from build123d import *

# Parameters (mm, degrees)
SKETCH1_W           = 300
SKETCH1_H           = 170
BOSS_EXTRUDE1_DEPTH = 12
SKETCH2_R           = 4
CUT_EXTRUDE1_DEPTH  = 13
SKETCH4_R           = 4
CUT_EXTRUDE2_DEPTH  = 13
SKETCH5_R           = 4
CUT_EXTRUDE3_DEPTH  = 13
SKETCH6_W           = 46.5
SKETCH6_H           = 93
SKETCH6_W_2         = 80
SKETCH6_H_2         = 45
SKETCH6_W_3         = 64
SKETCH6_H_3         = 67.5
SKETCH6_W_4         = 23.5
SKETCH6_H_4         = 65.5
CUT_EXTRUDE4_DEPTH  = 13
FILLET1_R           = 10


with BuildPart() as part:
    # Sketch1 → Boss-Extrude1 (new body)
    with BuildSketch(Plane(origin=(0, 0, 0), x_dir=(1, 0, 0), z_dir=(0, 1, 0))):
        Rectangle(SKETCH1_W, SKETCH1_H)
    extrude(amount=BOSS_EXTRUDE1_DEPTH)

    # Sketch2 → Cut-Extrude1 (cut, through all)
    with BuildSketch(Plane(origin=(0, 12, 0), x_dir=(1, 0, 0), z_dir=(0, 1, 0))):
        with Locations((-135, 65)):
            Circle(SKETCH2_R)
        with Locations((-135, 23)):
            Circle(SKETCH2_R)
        with Locations((-135, -19)):
            Circle(SKETCH2_R)
        with Locations((-135, -61)):
            Circle(SKETCH2_R)
        with Locations((-135, -103)):
            Circle(SKETCH2_R)
        with Locations((-135, -145)):
            Circle(SKETCH2_R)
    cut_extrude1 = extrude(amount=-CUT_EXTRUDE1_DEPTH, mode=Mode.SUBTRACT)

    # Mirror1: Cut-Extrude1 across plane
    add(cut_extrude1.mirror(Plane(origin=(0, 0, 0), x_dir=(0, 0, 1), z_dir=(1, 0, 0))), mode=Mode.SUBTRACT)

    # Sketch4 → Cut-Extrude2 (cut, through all)
    with BuildSketch(Plane(origin=(0, 12, 0), x_dir=(1, 0, 0), z_dir=(0, 1, 0))):
        with Locations((-110, 65)):
            Circle(SKETCH4_R)
        with Locations((-10, 65)):
            Circle(SKETCH4_R)
        with Locations((-110, 40)):
            Circle(SKETCH4_R)
        with Locations((-10, 40)):
            Circle(SKETCH4_R)
        with Locations((46, 65)):
            Circle(SKETCH4_R)
        with Locations((46, 15)):
            Circle(SKETCH4_R)
    extrude(amount=-CUT_EXTRUDE2_DEPTH, mode=Mode.SUBTRACT)

    # Sketch5 → Cut-Extrude3 (cut, through all)
    with BuildSketch(Plane(origin=(0, 12, 0), x_dir=(1, 0, 0), z_dir=(0, 1, 0))):
        with Locations((-60, -20)):
            Circle(SKETCH5_R)
        with Locations((-60, -50)):
            Circle(SKETCH5_R)
        with Locations((84, -20)):
            Circle(SKETCH5_R)
        with Locations((84, -50)):
            Circle(SKETCH5_R)
    extrude(amount=-CUT_EXTRUDE3_DEPTH, mode=Mode.SUBTRACT)

    # Sketch6 → Cut-Extrude4 (cut, through all)
    with BuildSketch(Plane(origin=(0, 12, 0), x_dir=(1, 0, 0), z_dir=(0, 1, 0))):
        with Locations((-100.75, -26.5)):
            Rectangle(SKETCH6_W, SKETCH6_H)
        Polygon((27.5, 20), (-42.5, 20), (-42.5, -73), (66.5, -73), (66.5, -7.5), (27.5, -7.5), align=None)
        with Locations((-60, 52.5)):
            Rectangle(SKETCH6_W_2, SKETCH6_H_2)
        with Locations((93, 41.25)):
            Rectangle(SKETCH6_W_3, SKETCH6_H_3)
        with Locations((113.25, -40.25)):
            Rectangle(SKETCH6_W_4, SKETCH6_H_4)
    extrude(amount=-CUT_EXTRUDE4_DEPTH, mode=Mode.SUBTRACT)

    # Fillet1
    fillet1_edges = [part.edges().sort_by_distance(p)[0] for p in [
        (-42.5, 6, 73),
        (-42.5, 6, -20),
        (27.5, 6, -20),
        (27.5, 6, 7.5),
        (66.5, 6, 7.5),
        (66.5, 6, 73),
        (-20, 6, -75),
        (-20, 6, -30),
        (-100, 6, -30),
        (-100, 6, -75),
        (125, 6, -75),
        (125, 6, -7.5),
        (61, 6, -7.5),
        (61, 6, -75),
        (125, 6, 7.5),
        (125, 6, 73),
        (101.5, 6, 73),
        (101.5, 6, 7.5),
        (-124, 6, 73),
        (-124, 6, -20),
        (-77.5, 6, -20),
        (-77.5, 6, 73),
    ]]
    fillet(fillet1_edges, radius=FILLET1_R)


solid = part.part
Verification items for the finished model (mm, model axes). Give positions to 0.01 mm unless a question says otherwise; leave off trailing zeros. Write each loop counter-clockwise with the first axis right and the second up, starting at its lowest first coordinate (ties: lowest second). Pieces come first, ordered by that corner, then holes.
(1) Cross-section at C-C (z = -23). Enter the section's corners in (x, y), plus the area to 3 significant figures.
(2) Gauge pin test, flat end, axial feed: pin 1 (9 mm diameter, centred on x = 46, z = -15, fed in from -Y). Record the tip position at first contact, or that the pin passes through.
(3) Material ranges on line 1 (X direction, y = 8.5, z = 50); line 2 (Z direction, x = -60, y = 9); line 3 (X direction, y = 9.75, z = -7), recorded low to high.
(4) Cross-section at D-D (x = -97). Enter the section's corners in (y, z).
(5) Cross-section at B-B (x = 46). Enter the section's corners in (y, z), plus the area to 3 significant figures.
(6) Cross-section at A-A (z = 50). Enter the section's corners in (x, y), plus the area to 3 significant figures.
(7) Mould release check, pull along Z, two halves, no side actions. Record for faces 1 (the face through (-2, 6, 85)), 2 (the face through (-131.185, 6.084, 17.799)), 3 (the face through (31, 12, -1)): +Z half, -Z half, draft (parallel to the pull), parting line (faces both ways), or undercut.
Worked out:
1. outline: (-150, 0) - (-139, 0) - (-139, 12) - (-150, 12) - close; (-131, 0) - (61, 0) - (61, 12) - (-131, 12) - close; (125, 0) - (131, 0) - (131, 12) - (125, 12) - close; (139, 0) - (150, 0) - (150, 12) - (139, 12) - close
1. area: 2,640 mm2
2. pin 1: stops at y = 0
3. line 1: x = -150 to -124, -77.5 to -64, -56 to -42.5, 66.5 to 80, 88 to 101.5, 125 to 150
3. line 2: z = -85 to -75, -30 to 16, 24 to 46, 54 to 85
3. line 3: x = -150 to -124, -77.5 to -42.5, 27.5 to 150
4. outline: (0, -85) - (12, -85) - (12, -72.14) - (0, -72.14) - close; (0, -32.86) - (12, -32.86) - (12, -20) - (0, -20) - close; (0, 73) - (12, 73) - (12, 85) - (0, 85) - close
5. outline: (0, -85) - (12, -85) - (12, -69) - (0, -69) - close; (0, -61) - (12, -61) - (12, -19) - (0, -19) - close; (0, -11) - (12, -11) - (12, 7.5) - (0, 7.5) - close; (0, 73) - (12, 73) - (12, 85) - (0, 85) - close
5. area: 1,060 mm2
6. outline: (-150, 0) - (-124, 0) - (-124, 12) - (-150, 12) - close; (-77.5, 0) - (-64, 0) - (-64, 12) - (-77.5, 12) - close; (-56, 0) - (-42.5, 0) - (-42.5, 12) - (-56, 12) - close; (66.5, 0) - (80, 0) - (80, 12) - (66.5, 12) - close; (88, 0) - (101.5, 0) - (101.5, 12) - (88, 12) - close; (125, 0) - (150, 0) - (150, 12) - (125, 12) - close
6. area: 1,260 mm2
7. face 1: +Z half
7. face 2: undercut
7. face 3: draft
